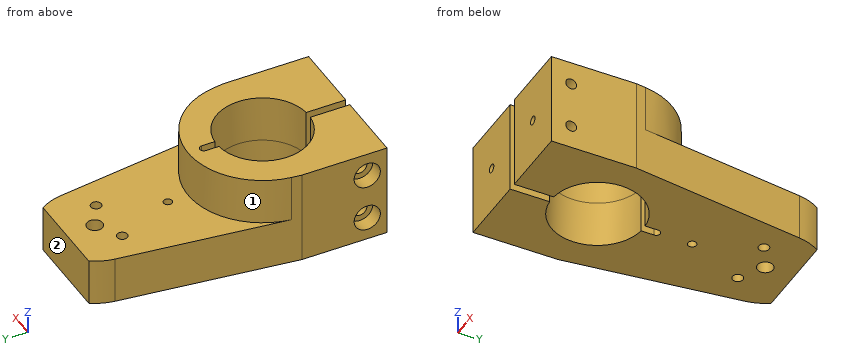
Autodesk Inventor part; units mm, degrees
ref_plane "YZ Plane" through (0, 0, 0) normal (1, 0, 0) x (0, 1, 0)
ref_plane "XZ Plane" through (0, 0, 0) normal (0, 1, 0) x (-1, 0, 0)
ref_plane "XY Plane" through (0, 0, 0) normal (0, 0, 1) x (1, 0, 0)
sketch "Skizze1" plane through (0, 0, 0) normal (0, 0, 1) x (1, 0, 0)
  circle A0 centre (0, 0) radius 20 construction
  line L0 (-19.8289, 2.6105) -> (-28.5983, -64)
  line L1 (19.8289, 2.6105) -> (28.5983, -64)
  circle A1 centre (0, 0) radius 11 construction
  line L2 (0, 0) -> (0, 20) construction
  line L3 (0, 0) -> (0, -96.5) construction
  circle A2 centre (0, -64) radius 17.5
  line L4 (-19.8289, 2.6105) -> (0, 153.226) construction
  line L5 (19.8289, 2.6105) -> (0, 153.226) construction
  circle A3 centre (0, 25) radius 80 construction
  circle A4 centre (0, -64) radius 6 construction
  arc A5 (19.8289, 2.6105) -> (-19.8289, 2.6105) centre (0, 0) ccw
  line L6 (28.5983, -64) -> (28.5983, -96.5)
  line L7 (28.5983, -96.5) -> (-28.5983, -96.5)
  line L8 (-28.5983, -96.5) -> (-28.5983, -64)
  line L9 (0, -64) -> (-28.5983, -64) construction
  line L10 (0, -89) -> (-28.5983, -89) construction
  line L11 (0, -86.5) -> (-28.5983, -86.5) construction
  line L12 (0, -91.5) -> (-28.5983, -91.5) construction
  line L13 (1.5, -64) -> (-1.5, -64)
  line L14 (-1.5, -64) -> (-1.5, -96.5)
  line L15 (-1.5, -96.5) -> (1.5, -96.5)
  line L16 (1.5, -96.5) -> (1.5, -64)
  line L17 (-16.7033, 11) -> (16.7033, 11)
  circle A6 centre (0, 0) radius 3
  line L18 (-1.5, -46.5644) -> (-1.5, -41.5644)
  arc A7 (1.5, -41.5644) -> (-1.5, -41.5644) centre (0, -41.5644) ccw
  line L19 (1.5, -41.5644) -> (1.5, -46.5644)
  line L20 (1.5, -46.5644) -> (-1.5, -46.5644)
  point P0 (0, 11)
  point P1 (-9.5263, -5.5)
  point P2 (9.5263, -5.5)
  point P3 (0, -55)
  point P4 (0, -58)
  point P5 (0, -46.5)
  point P6 (0, -81.5)
  point P7 (-1.5, -81.4356)
  point P8 (1.5, -81.4356)
  point P9 (0, -46.5644)
  dimension "d9" = 22
  dimension "d54" = 160
  dimension "d56" = 12
  dimension "d2" = 360
  dimension "d10" = 40
  dimension "d47" = 25
  dimension "d51" = 3
  dimension "d52" = 15
  dimension "d55" = 35
  dimension "d61" = 5
  dimension "d62" = 2.5
  dimension "d63" = 5
  dimension "d65" = 3
  dimension "d66" = 5
  dimension "d81" = 11
  dimension "d82" = 6
  dimension "d85" = 3
  dimension "d86" = 5
extrude "Extrusion1" add sketch "Skizze1" along normal blind 18 contours A5 L17 L1 L6 L7 L16 A2 L19 A7 L18 L14 L8 L0
hole "Bohrung1" at (-9.5263, -5.5, 0) at (9.5263, -5.5, 0) direction (0, 0, 1) diameter 4 end through all
sketch "Skizze4" plane through (0, 0, 18) normal (0, 0, 1) x (1, 0, 0)
  circle A0 centre (0, -64) radius 28.3537
  line L0 (28.5983, -64) -> (19.8289, 2.6105)
  line L1 (-28.5983, -64) -> (-28.5983, -96.5)
  line L2 (-19.8289, 2.6105) -> (-28.5983, -64)
  line L3 (28.5983, -96.5) -> (28.5983, -64)
  line L4 (1.5, -96.5) -> (28.5983, -96.5)
  line L5 (-28.5983, -96.5) -> (-1.5, -96.5)
  line L6 (-1.5, -96.5) -> (-1.5, -81.4356)
  arc A1 (1.5, -81.4356) -> (-1.5, -81.4356) centre (0, -64) ccw
  line L7 (1.5, -81.4356) -> (1.5, -96.5)
  line L8 (1.5, -96.5) -> (1.5, -81.4356)
  line L9 (-1.5, -46.5644) -> (-1.5, -41.5644)
  arc A2 (1.5, -41.5644) -> (-1.5, -41.5644) centre (0, -41.5644) ccw
  line L10 (1.5, -41.5644) -> (1.5, -46.5644)
  line L11 (1.5, -46.5644) -> (-1.5, -46.5644)
  point P0 (0, 0)
  point P1 (28.1111, -60.2991)
  point P2 (-28.1111, -60.2991)
extrude "Extrusion2" add sketch "Skizze4" along normal blind 18 contours A0 L7 A1 L10 A2 L9 L6 | A0 L0 L3 L4 L7 | A0 L6 L5 L1 L2
ref_plane "Arbeitsebene1" through (0, 0, 18) normal (0, 0, 1) x (1, 0, 0)
sketch "Skizze2" plane through (1.5, -96.5, 0) normal (-1, 0, 0) x (0, 0, 1)
  line L0 (0, 15.0644) -> (0, 0) construction
  line L1 (0, 0) -> (36, 0) construction
  line L2 (0, 15.0644) -> (36, 15.0644) construction
  line L3 (0, 0) -> (18, 0) construction
  line L4 (0, 15.0644) -> (18, 0) construction
  line L5 (18, 15.0644) -> (0, 0) construction
  line L6 (36, 15.0644) -> (36, 0)
  line L7 (18, 129) -> (18, -21.5) construction
  point P0 (0, 96.5)
  point P1 (9, 7.5322)
  point P2 (27, 7.5322)
hole "Bohrung3" at (1.5, -88.9678, 9) at (1.5, -88.9678, 27) direction (1, 0, 0) diameter 4.134 end through all
sketch "Skizze3" plane through (-28.5983, -96.5, 0) normal (-1, 0, 0) x (0, 0, 1)
  point P0 (0, 96.5)
  point P1 (9, 7.5322)
  point P2 (27, 7.5322)
hole "Bohrung4" at (-28.5983, -88.9678, 9) at (-28.5983, -88.9678, 27) direction (1, 0, 0) diameter 5.5 depth 27.0983 counterbore diameter 10 counterbore depth 5.5
sketch "Skizze5" plane through (1.5, -96.5, 0) normal (0, -1, 0) x (1, 0, 0)
  line L0 (38.5377, 27) -> (-41.5377, 27) construction
  line L1 (38.5377, 9) -> (-41.5377, 9) construction
  line L2 (-41.5377, 18) -> (38.5377, 18) construction
  line L3 (-3, 36) -> (0, 36) construction
  line L4 (-1.5, 36) -> (-1.5, 0) construction
  point P0 (13.5, 18)
  point P1 (-16.5, 18)
  dimension "d87" = 15
  dimension "d88" = 30
hole "Bohrung5" at (15, -96.5, 18) at (-15, -96.5, 18) direction (0, 1, 0) diameter 3.242 depth 11.8 tip angle 118
sketch "Skizze6" plane through (0, 0, 0) normal (0, 0, -1) x (-1, 0, 0)
  arc A0 (28.1111, -60.2991) -> (-28.1111, -60.2991) centre (0, -64) ccw construction
  line L0 (0, 0) -> (0, -96.5) construction
  circle A1 centre (0, 0) radius 20 construction
  point P0 (0, -27.8963)
  point P1 (0, -20)
  point P2 (0, -35.6463)
  dimension "d96" = 15.6463
  dimension "d97" = 7.75
hole "Bohrung6" at (0, -27.8963, 0) direction (0, 0, 1) diameter 3.242 end through all
equation "\"d9\" = FixationHole_Dia"
equation "\"d10\" = MotrGC_Part_OuterDia"
properties part number "GC_Motor_Aussenscheibe" material "PBT-Kunststoff"
Model file for the job. Use its own axes, mm. Face numbers are marked on the shaded views. A direction names the side the tool comes from. Give positions to 0.01 mm unless a question says otherwise; leave off trailing zeros. Order: outer loops, then holes, each group sorted by start corner. A loop starts at its lowest first (then second) coordinate and runs counter-clockwise, first axis right, second up. Notation, with made-up numbers: M 58,38 L 102,38 A7 cw 102,51 Z; hole C 48.25,63.5 d9. An arc over 180 degrees is marked long. Put each result on its own line as item: value. Start each with the question number.
(1) Pin check, flat tips, straight feed: pin 1 Ø3 at (x, y) = (-1, -24.5) entering from +Z; pin 2 Ø3 at (x, z) = (15, 18) entering from -Y; pin 3 Ø4 at (y, z) = (-45, 21) entering from +X. Stop position of each tip, or through.
(2) Band-saw the part on C-C on y = -5.5. Give the cut face in (x, z).
(3) Band-saw the part on A-A on x = 0. Give the cut face in (y, z), then the cut area to 3 significant figures.
(4) Tool access for the marked faces 1 and 2: list every direction of +Z, -Z, +X, -X, +Y, -Y with a clear straight run to the whole face (end or side of a thin tool).
(5) Drill centre lines: L1, parallel to Y at x = 0, z = 14; L2, parallel to X at y = -87.5, z = 23; L3, parallel to Y at x = 13.5, z = 27. Where is each one in solid material? Low to high. Write a range as [from, to].
(6) Band-saw the part on B-B on z = 9. Count the separate pieces of the cut face and the enclosed holes in it, then the cut area to 3 significant figures.
(7) Band-saw the part on D-D on x = 6. Give the cut face in (y, z).
Results below:
1. pin 1: stops at z = 18
1. pin 2: stops at y = -84.63
1. pin 3: stops at x = 22.69
2. outline: M -20.9,0 L -11.53,0 L -11.53,18 L -20.9,18 Z; M -7.53,0 L 7.53,0 L 7.53,18 L -7.53,18 Z; M 11.53,0 L 20.9,0 L 20.9,18 L 11.53,18 Z
3. outline: M -40.06,0 L -29.52,0 L -29.52,18 L -35.65,18 L -35.65,36 L -40.06,36 Z; M -26.28,0 L -3,0 L -3,18 L -26.28,18 Z; M 3,0 L 11,0 L 11,18 L 3,18 Z
3. area: 832 mm2
4. face 1: +Z, +Y
4. face 2: +Z, -Z, +X, -X, +Y
5. L1: y = [-40.06, -29.52], [-26.28, -3], [3, 11]
5. L2: x = [-23.1, -1.5], [1.5, 28.6]
5. L3: y = [-96.5, -91.03], [-86.9, -75.14], [-52.86, -39.07]
6. separate pieces: 3
6. enclosed holes: 4
6. area: 4,020 mm2
7. outline: M -96.5,0 L -80.44,0 L -80.44,36 L -96.5,36 Z; M -47.56,0 L 11,0 L 11,18 L -36.29,18 L -36.29,36 L -47.56,36 Z; hole C -88.97,9 d4.13; hole C -88.97,27 d4.13
